The model under review builds one solid part; all positions refer to its coordinate system, in mm. A direction names the side the tool comes from. Round coordinates to 2 decimals unless told otherwise and drop trailing zeros. Write each loop counter-clockwise with the first axis right and the second up, starting at its lowest first coordinate (ties: lowest second). Pieces come first, ordered by that corner, then holes. Notation, with made-up numbers: (-3, -3.75) -> (28, -3.75) arc R32 cw to (28, 27.25) -> close; hole circle Ø8 at (25, -3.75). An arc over 180 degrees is marked (long way). Return JSON: item names as keys, results as strings. Group by question number.
1. Take a section at A-A, the plane x = 89. Write out the cut boundary in (y, z).
2. For line 1 along Z through (x, y) = (-1.5, 2.75); line 2 along Z through (x, y) = (2.5, 1.5); line 3 along Z through (x, y) = (22, -2.5), list the stretches that pass through material, from the lowest coordinate up. Write a range as from..to.
3. Clearance check with flat-ended pins moving along their axes: P1, Ø1.5, axis at x = 96.5, y = -3.5, coming from the -Z side; P2, Ø4, axis at x = 76, y = 0.5, coming from the +Z side; P3, Ø5, axis at y = 0.5, z = 8, coming from the +X side. State where each tip first meets the part, or that it passes through.
4. Mouldability with a two-part tool opening along X and no side actions: class faces 4 (the cylindrical face through (11.97, 0.07, 98.19)), 5 (the cylindrical face through (-9.853, 0.07, -99.73)), 6 (the cylindrical face through (93.38, 0.07, -29.9)) as pulls with the +X half, pulls with the -X half, needs draft (parallel to the pull), parting line crosses it, or undercut.
5. Take a section at C-C, the plane y = 0. Write out the cut boundary in (x, z).
6. Take a section at B-B, the plane z = -94.3. Write out the cut boundary in (x, y).
7. Take a section at D-D, the plane z = 32.5. Write out the cut boundary in (x, y).
8. Tool access review of faces 1 (the cylindrical face through (105.776, 0.07, 6.575)), 2 (the cylindrical face through (38.532, 0.07, -90.161)), 3 (the flat face through (84, -5, -9)): name each direction out of +Z, -Z, +X, -X, +Y, -Y from which nothing blocks a thin tool from reaching the whole face with its end or side.
from build123d import *

# Parameters (mm, degrees)
BOSS_EXTRUDE1_DEPTH  = 5
M5_CLEARANCE_HOLE1_D = 5.5
FILLET1_R            = 10


with BuildPart() as part:
    # Sketch1 → Boss-Extrude1 (new, symmetric)
    with BuildSketch(Plane(origin=(0, 0, 0), x_dir=(1, 0, 0), z_dir=(0, 1, 0))):
        with BuildLine():
            ThreePointArc((115.470324267, -24.543975101), (112.272221749, 36.479456186), (78.990868081, 87.728246648))
            Line((78.990868081, 87.728246648), (65.608255953, 72.865350138))
            ThreePointArc((65.608255953, 72.865350138), (40.133036877, 89.460280857), (10.798978706, 97.45349947))
            ThreePointArc((10.798978706, 97.45349947), (-9.001093518, 101.04854173), (0, 83.05))
            ThreePointArc((0, 83.05), (83.05, 0), (0, -83.05))
            ThreePointArc((0, -83.05), (-9.001093518, -101.04854173), (10.798978706, -97.45349947))
            ThreePointArc((10.798978706, -97.45349947), (65.813533347, -72.679992628), (95.907372252, -20.385741285))
            Line((95.907372252, -20.385741285), (115.470324267, -24.543975101))
        make_face()
        with BuildLine():
            ThreePointArc((113.045695402, 0.986534838), (105.611429996, -6.578628601), (98.046266556, 0.855636806))
            ThreePointArc((98.046266556, 0.855636806), (93.251091423, 30.299116298), (79.824026575, 56.937924807))
            ThreePointArc((79.824026575, 56.937924807), (81.574620795, 67.399063363), (92.03575935, 65.648469143))
            ThreePointArc((92.03575935, 65.648469143), (107.516939167, 34.934371214), (113.045695402, 0.986534838))
        make_face(mode=Mode.SUBTRACT)
    extrude(amount=BOSS_EXTRUDE1_DEPTH, both=True)

    # M5 Clearance Hole1 (through all)
    with Locations(Plane(origin=(0, 5, 0), x_dir=(1, 0, 0), z_dir=(0, 1, 0))):
        with Locations((0, -94.3), (0, 94.3)):
            Hole(M5_CLEARANCE_HOLE1_D / 2)

    # Fillet1
    # the kernel refuses this fillet: 10 mm, written as the material it adds along each edge
    with BuildSketch(Plane(origin=(10.798978706, 5, 97.45349947), x_dir=(0.990831071127436, 0, -0.13510658195831074), z_dir=(0, -1, 0)), Plane(origin=(10.798978706, -5, -97.45349947), x_dir=(0.990831071127436, 0, 0.13510658195831213), z_dir=(0, 1, 0))) as fillet1_piece_1:
        with BuildLine():
            CenterArc((5.184861326, 9.996835122), FILLET1_R, 223.325173882, 45.233283105)
            ThreePointArc((-2.089852288, 3.13545466), (-0.912718127, 1.655846999), (0, 0))
            ThreePointArc((0, 0), (2.466645575, 0.031031634), (4.93329115, 0))
        make_face()
    extrude(amount=10)
    with BuildSketch(Plane(origin=(65.608255953, -5, -72.865350138), x_dir=(0.6691306063588537, 0, -0.7431448254773984), z_dir=(0, 1, 0)), Plane(origin=(95.907372252, 5, 20.385741285), x_dir=(0.9781476007338056, 0, 0.20791169081775965), z_dir=(0, -1, 0))) as fillet1_piece_2:
        with BuildLine():
            CenterArc((9.536256092, 10), FILLET1_R, 185.31030916, 84.68969084)
            ThreePointArc((-0.420824527, 9.074502545), (-0.105262635, 4.542127523), (0, 0))
            Line((0, 0), (9.536256092, 0))
        make_face()
    extrude(amount=10)
    # the kernel refuses this fillet: 10 mm, written as the material it takes off along each edge
    with BuildSketch(Plane(origin=(78.990868081, -32.343098115, -87.728246648), x_dir=(0.7113498032891118, 0, 0.7028381444973957), z_dir=(0, 1, 0))) as fillet1_2_piece_1:
        with BuildLine():
            CenterArc((10.473993196, -9.989264392), FILLET1_R, 87.34484542, 95.31030916)
            Line((0.484728804, -10.452510442), (0, 0))
            ThreePointArc((0, 0), (5.468619623, 0.12673385), (10.937239246, 0))
        make_face()
    extrude(amount=64.68619623, mode=Mode.SUBTRACT)
    with BuildSketch(Plane(origin=(115.470324267, -32.343098115, 24.543975101), x_dir=(-0.9781476007338059, 0, -0.2079116908177584), z_dir=(0, 1, 0))) as fillet1_2_piece_2:
        with BuildLine():
            CenterArc((10.463743908, -10), FILLET1_R, 90, 95.31030916)
            ThreePointArc((0.506663288, -10.925497455), (0.12673385, -5.468619623), (0, 0))
            Line((0, 0), (10.463743908, 0))
        make_face()
    extrude(amount=64.68619623, mode=Mode.SUBTRACT)


solid = part.part
Output:
{
 "1": {"outline": "(-5, -77.56) -> (5, -77.56) -> (5, -68.14) -> (-5, -68.14) -> close; (-5, -41.14) -> (5, -41.14) -> (5, 41.14) -> (-5, 41.14) -> close"},
 "2": {"line 1": "z = -105.45..-96.6, -92..-83.15, 83.15..92, 96.6..105.45", "line 2": "z = -105.27..-95.45, -93.15..-83.01, 83.01..93.15, 95.45..105.27", "line 3": "z = -95.55..-80.08, 80.08..95.55"},
 "3": {"P1": "stops at z = -69.05", "P2": "stops at z = 64.33", "P3": "stops at x = 117.92"},
 "4": {"face 4": "pulls with the +X half", "face 5": "parting line crosses it", "face 6": "undercut"},
 "5": {"outline": "(0, -83.05) arc R11.25 ccw (long way) to (9.15, -100.84) arc R10 cw to (15.69, -96.79) arc R98.05 ccw to (58.58, -78.62) arc R10 cw to (71.99, -79.95) arc R10 ccw to (86.77, -80.04) arc R118.05 ccw to (117.25, 13.75) arc R10 ccw to (105.24, 22.37) arc R10 cw to (93.61, 29.17) arc R98.05 ccw to (15.69, 96.79) arc R10 cw to (9.15, 100.84) arc R11.25 ccw (long way) to (0, 83.05) arc R83.05 cw to start; hole circle Ø5.5 at (0, -94.3); hole circle Ø5.5 at (0, 94.3); hole (79.82, -56.94) arc R7.5 ccw to (92.04, -65.65) arc R113.05 ccw to (113.05, -0.99) arc R7.5 ccw to (98.05, -0.86) arc R98.05 cw to start"},
 "6": {"outline": "(-11.25, -5) -> (-2.75, -5) -> (-2.75, 5) -> (-11.25, 5) -> close; (2.75, -5) -> (26.86, -5) -> (26.86, 5) -> (2.75, 5) -> close"},
 "7": {"outline": "(76.43, -5) -> (92.51, -5) -> (92.51, 5) -> (76.43, 5) -> close"},
 "8": {"face 1": "+Y, -Y", "face 2": "-Z, +Y, -Y", "face 3": "+Z, -Z, +X, -X, -Y"}
}
